from build123d import *

# Parameters (mm, degrees)
SKICA1_R                = 0.5
P_IDAT_VYSUNUT_M1_DEPTH = 2


with BuildPart() as part:
    # Skica1 → Přidat vysunutím1 (new body)
    with BuildSketch(Plane.XY):
        with BuildLine():
            Line((0, 11), (0, 12))
            Line((0, 12), (-48.307823831, 12))
            ThreePointArc((-48.307823831, 12), (-49.570592062, 11.550940487), (-50.266302206, 10.405416394))
            ThreePointArc((-50.266302206, 10.405416394), (-51.024263074, 5.612344033), (-51.326233925, 0.769115673))
            ThreePointArc((-51.326233925, 0.769115673), (-51.324464931, 0.649874315), (-51.31559221, 0.530950366))
            ThreePointArc((-51.31559221, 0.530950366), (-26.186308465, 8.356056534), (0, 11))
        make_face()
        with Locations((-45.246630015, 5.5)):
            Circle(SKICA1_R, mode=Mode.SUBTRACT)
    extrude(amount=P_IDAT_VYSUNUT_M1_DEPTH)


solid = part.part
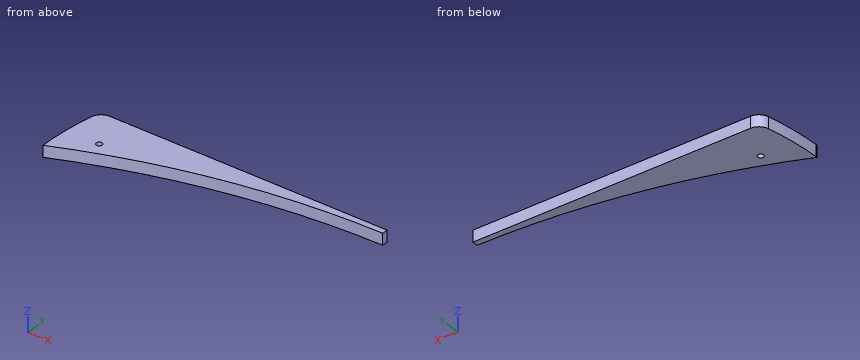
Part model, mm, in its own coordinate system. Give positions to 0.01 mm unless a question says otherwise; leave off trailing zeros. Loops run counter-clockwise (first coordinate to the right, second up) from the corner with the lowest first, then second, coordinate; pieces in that order, holes last.
(1) Pin check, flat tip, straight feed: pin 1 (1 mm diameter, centred on x = -37, z = 1.5, fed in from -Y). Stop position of the tip, or through.
Return value:
pin 1: stops at y = 5.52
(2) Band-saw the part on D-D (y = 2.5). Write the cut outline in (x, z).
Return value:
outline: (-51.27, 0) - (-46.42, 0) - (-46.42, 2) - (-51.27, 2) - close
(3) Band-saw the part on C-C (x = -47). Write the cut outline in (y, z), and give its area (3 significant figures).
Return value:
outline: (2.28, 0) - (12, 0) - (12, 2) - (2.28, 2) - close
area: 19.4 mm2
(4) Band-saw the part on A-A (y = 5.5). Write the cut outline in (x, z), and give its area (3 significant figures).
Return value:
outline: (-51.04, 0) - (-45.75, 0) - (-45.75, 2) - (-51.04, 2) - close; (-44.75, 0) - (-37.56, 0) - (-37.56, 2) - (-44.75, 2) - close
area: 25.0 mm2
(5) Drill centre lines: line 1 along Y through (x, z) = (-13.5, 0.45); line 2 along Y through (x, z) = (-17, 0.35); line 3 along X through (y, z) = (1.25, 1.35). Where is each one in solid material? Low to high.
Return value:
line 1: y = 10.3 to 12
line 2: y = 9.89 to 12
line 3: x = -51.32 to -49.59
(6) Band-saw the part on B-B (z = 1). Write the cut outline in (x, y), and give its area (3 significant figures).
Return value:
outline: (-51.33, 0.77) arc R2 ccw to (-51.32, 0.53) arc R131 cw to (0, 11) - (0, 12) - (-48.31, 12) arc R2 ccw to (-50.27, 10.41) arc R51.33 ccw to start; hole circle Ø1 at (-45.25, 5.5)
area: 221 mm2
